Verification items for the finished model (mm, model axes). Face numbers are marked on the shaded views. Coordinates: 2 decimals unless noted, no trailing zeros. Order: outer loops, then holes, each group sorted by start corner. A loop starts at its lowest first (then second) coordinate and runs counter-clockwise, first axis right, second up. Notation, with made-up numbers: M 50,-33 L 82,-33 A25 cw 82,-16 Z; hole C 36.5,4 d5. An arc over 180 degrees is marked long. Return JSON: item names as keys, results as strings. Group by question number.
Q1. Mould release check, pull along Z, two halves, no side actions. Record for the marked faces 1 and 2: pulls with the +Z half, pulls with the -Z half, needs draft (parallel to the pull), parting line crosses it, or undercut.
Q2. Section check D-D, the plane y = 20. Enter the section's corners in (x, z), then the cut area to 3 significant figures.
Q3. Go/stop test with flat-tipped pins: pin 1 Ø3 at (x, y) = (-10.5, 25.5) entering from -Z; pin 2 Ø12 at (y, z) = (18, -10.5) entering from -X; pin 3 Ø1.5 at (y, z) = (8, 52) entering from -X. Record where each tip stops, or that it passes through.
Q4. Section check B-B, the plane x = -14.5. Enter the section's corners in (y, z).
Q5. Thickness scan on probe 1 along Z at (x, y) = (-4.5, 27); probe 2 along Z at (x, y) = (-91, 13.25); probe 3 along X at (y, z) = (27, 13.5). Record the ranges inside material, lowest first.
Q6. Section check C-C, the plane z = 0. Enter the section's corners in (x, y), then the cut area to 3 significant figures.
Autodesk Inventor part; units mm, degrees
ref_plane "YZ Plane" through (0, 0, 0) normal (1, 0, 0) x (0, 1, 0)
ref_plane "XZ Plane" through (0, 0, 0) normal (0, 1, 0) x (-1, 0, 0)
ref_plane "XY Plane" through (0, 0, 0) normal (0, 0, 1) x (1, 0, 0)
sketch "Sketch1" plane through (0, 0, 0) normal (0, 1, 0) x (-1, 0, 0)
  circle A0 centre (0, 0) radius 100
  circle A1 centre (0, 0) radius 103
  line L0 (0, -100) -> (0, -103)
  line L1 (0, 100) -> (0, 103)
  point P0 (0, 101.5)
  dimension "d0" = 200
  dimension "d1" = 206
extrude "Extrusion1" add sketch "Sketch1" along normal blind 30 contours A0 L1 A1 L0 picked at (101.4211, -8.8323)
properties part number "R10_CM_CIRCULO"
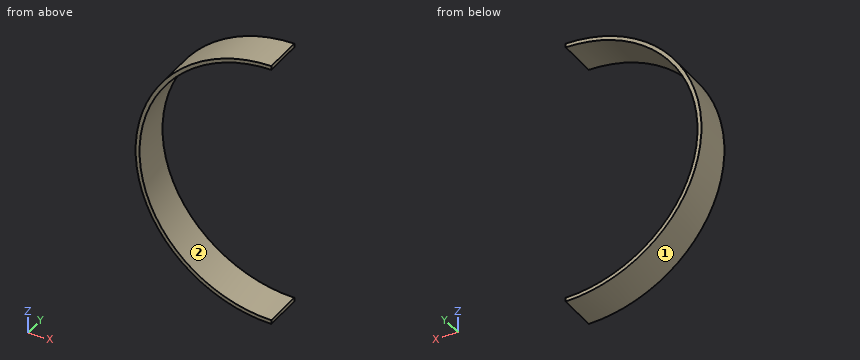
Numbers:
{
 "1": {"face 1": "parting line crosses it", "face 2": "undercut"},
 "2": {"outline": "M 0,-103 L 0,-100 A100 cw 0,100 L 0,103 A103 ccw Z", "area": "957 mm2"},
 "3": {"pin 1": "stops at z = -102.61", "pin 2": "stops at x = -102.9", "pin 3": "stops at x = -89.34"},
 "4": {"outline": "M 0,-101.97 L 30,-101.97 L 30,-98.94 L 0,-98.94 Z; M 0,98.94 L 30,98.94 L 30,101.97 L 0,101.97 Z"},
 "5": {"probe 1": "z = -102.9 to -99.9, 99.9 to 102.9", "probe 2": "z = -48.25 to -41.46, 41.46 to 48.25", "probe 3": "x = -102.11 to -99.08"},
 "6": {"outline": "M -103,0 L -100,0 L -100,30 L -103,30 Z", "area": "90.0 mm2"}
}
